Part model, mm, in its own coordinate system. A direction names the side the tool comes from. Round coordinates to 2 decimals unless told otherwise and drop trailing zeros. Loops run counter-clockwise (first coordinate to the right, second up) from the corner with the lowest first, then second, coordinate; pieces in that order, holes last.
(1) Mould opens along X. For faces 1 (the face through (92.5, -51.5, -4.8)), 2 (the face through (-96.343, -55.072, -5.916)), 3 (the face through (96.343, 55.072, -5.916)) say: +X half, -X half, draft (parallel to the pull), parting line (faces both ways), or undercut.
(2) Tool access for faces 4 (the face through (-74, -38, -11.4)), 5 (the face through (57.83, -29.62, -11.7)), 6 (the face through (96.172, -55.243, -5.916)): list every direction of +Z, -Z, +X, -X, +Y, -Y with a clear straight run to the whole face (end or side of a thin tool).
(3) Flat gauge pins, fed straight in: pin 1 (0.5 mm diameter, centred on y = -48, z = -12, fed in from -X); pin 2 (7.5 mm diameter, centred on x = -76.5, y = -40, fed in from +Z). Where does each tip first touch, or does it go through?
(4) Cut at D-D on y = 33.8. List the corners of the cut face in (x, z) (3 decimals), then the cut area to 3 significant figures.
(5) Cut at A-A on y = 9.5. List the corners of the cut face in (x, z) (3 decimals).
(6) Cut at B-B on z = -4.75. List the corners of the cut face in (x, y).
(7) Probe probe 1 along X at (y, z) = (-16.5, -5); probe 2 along Y at (x, z) = (-63.1, -11.6) (3 decimals); probe 3 along Y at (x, z) = (83, -8). List the from-to ranges inside material, lowest first.
(8) Cut at C-C on x = -33.5. List the corners of the cut face in (y, z) (3 decimals).
Autodesk Inventor part; units mm, degrees
ref_plane "YZ Plane" through (0, 0, 0) normal (1, 0, 0) x (0, 1, 0)
ref_plane "XZ Plane" through (0, 0, 0) normal (0, 1, 0) x (-1, 0, 0)
ref_plane "XY Plane" through (0, 0, 0) normal (0, 0, 1) x (1, 0, 0)
sketch "Sketch1" plane through (0, 0, 0) normal (0, 0, 1) x (1, 0, 0)
  line L0 (77.5, 43.5) -> (77.5, -43.5)
  line L1 (77.5, -43.5) -> (-77.5, -43.5)
  line L2 (-77.5, -43.5) -> (-77.5, 43.5)
  line L3 (-77.5, 43.5) -> (77.5, 43.5)
  line L4 (85.48, 55.38) -> (-85.48, 55.38)
  arc A0 (-85.48, 55.38) -> (-96.48, 44.38) centre (-85.48, 44.38) ccw
  line L5 (-96.48, 44.38) -> (-96.48, -44.38)
  arc A1 (-96.48, -44.38) -> (-85.48, -55.38) centre (-85.48, -44.38) ccw
  line L6 (-85.48, -55.38) -> (85.48, -55.38)
  arc A2 (85.48, -55.38) -> (96.48, -44.38) centre (85.48, -44.38) ccw
  line L7 (96.48, -44.38) -> (96.48, 44.38)
  arc A3 (96.48, 44.38) -> (85.48, 55.38) centre (85.48, 44.38) ccw
  line L8 (-88.48, 58.38) -> (88.48, 58.38)
  line L9 (99.48, 47.38) -> (99.48, -47.38)
  line L10 (88.48, -58.38) -> (-88.48, -58.38)
  line L11 (-99.48, -47.38) -> (-99.48, 47.38)
  arc A4 (-88.48, 58.38) -> (-99.48, 47.38) centre (-88.48, 47.38) ccw
  arc A5 (99.48, 47.38) -> (88.48, 58.38) centre (88.48, 47.38) ccw
  arc A6 (88.48, -58.38) -> (99.48, -47.38) centre (88.48, -47.38) ccw
  arc A7 (-99.48, -47.38) -> (-88.48, -58.38) centre (-88.48, -47.38) ccw
  point P0 (0, 0)
  dimension "d0" = 3
  dimension "d1" = 3
  dimension "d2" = 3
  dimension "d3" = 3
  dimension "d4" = 11
  dimension "d5" = 11
extrude "Extrusion1" add sketch "Sketch1" against normal blind 12 contours L0 L1 L2 L3 | A3 L7 A2 L6 A1 L5 A0 L4 | L8 A5 L9 A6 L10 A7 L11 A4
sketch "Sketch2" plane through (0, 0, 0) normal (0, 0, 1) x (1, 0, 0)
  line L0 (-88.48, 58.38) -> (88.48, 58.38)
  arc A0 (-88.48, 58.38) -> (-99.48, 47.38) centre (-88.48, 47.38) ccw
  line L1 (-99.48, -47.38) -> (-99.48, 47.38)
  arc A1 (-99.48, -47.38) -> (-88.48, -58.38) centre (-88.48, -47.38) ccw
  line L2 (88.48, -58.38) -> (-88.48, -58.38)
  arc A2 (88.48, -58.38) -> (99.48, -47.38) centre (88.48, -47.38) ccw
  line L3 (99.48, 47.38) -> (99.48, -47.38)
  arc A3 (99.48, 47.38) -> (88.48, 58.38) centre (88.48, 47.38) ccw
  line L4 (77.5, 43.5) -> (77.5, -43.5)
  line L5 (77.5, -43.5) -> (-77.5, -43.5)
  line L6 (-77.5, -43.5) -> (-77.5, 43.5)
  line L7 (-77.5, 43.5) -> (77.5, 43.5)
  line L8 (85.48, 55.38) -> (-85.48, 55.38)
  arc A4 (-85.48, 55.38) -> (-96.48, 44.38) centre (-85.48, 44.38) ccw
  line L9 (-96.48, 44.38) -> (-96.48, -44.38)
  arc A5 (-96.48, -44.38) -> (-85.48, -55.38) centre (-85.48, -44.38) ccw
  line L10 (-85.48, -55.38) -> (85.48, -55.38)
  arc A6 (85.48, -55.38) -> (96.48, -44.38) centre (85.48, -44.38) ccw
  line L11 (96.48, -44.38) -> (96.48, 44.38)
  arc A7 (96.48, 44.38) -> (85.48, 55.38) centre (85.48, 44.38) ccw
  arc A8 (-85.48, 56.38) -> (-97.48, 44.38) centre (-85.48, 44.38) ccw
  line L12 (-85.48, 56.38) -> (85.48, 56.38)
  arc A9 (97.48, 44.38) -> (85.48, 56.38) centre (85.48, 44.38) ccw
  line L13 (97.48, 44.38) -> (97.48, -44.38)
  arc A10 (85.48, -56.38) -> (97.48, -44.38) centre (85.48, -44.38) ccw
  line L14 (85.48, -56.38) -> (-85.48, -56.38)
  arc A11 (-97.48, -44.38) -> (-85.48, -56.38) centre (-85.48, -44.38) ccw
  line L15 (-97.48, -44.38) -> (-97.48, 44.38)
  point P0 (0, 0)
  dimension "d8" = 1
extrude "Extrusion2" cut sketch "Sketch2" against normal blind 1.5 contours L4 L5 L6 L7 | A7 L11 A6 L10 A5 L9 A4 L8 | L12 A9 L13 A10 L14 A11 L15 A8
sketch "Sketch3" plane through (0, 0, -1.5) normal (0, 0, 1) x (1, 0, 0)
  arc A0 (-85.48, 56.38) -> (-97.48, 44.38) centre (-85.48, 44.38) ccw
  line L0 (-97.48, -44.38) -> (-97.48, 44.38)
  arc A1 (-97.48, -44.38) -> (-85.48, -56.38) centre (-85.48, -44.38) ccw
  line L1 (85.48, -56.38) -> (-85.48, -56.38)
  arc A2 (85.48, -56.38) -> (97.48, -44.38) centre (85.48, -44.38) ccw
  line L2 (97.48, 44.38) -> (97.48, -44.38)
  arc A3 (97.48, 44.38) -> (85.48, 56.38) centre (85.48, 44.38) ccw
  line L3 (-85.48, 56.38) -> (85.48, 56.38)
  arc A4 (-85.48, 54.38) -> (-95.48, 44.38) centre (-85.48, 44.38) ccw
  line L4 (-85.48, 54.38) -> (85.48, 54.38)
  arc A5 (95.48, 44.38) -> (85.48, 54.38) centre (85.48, 44.38) ccw
  line L5 (95.48, 44.38) -> (95.48, -44.38)
  arc A6 (85.48, -54.38) -> (95.48, -44.38) centre (85.48, -44.38) ccw
  line L6 (85.48, -54.38) -> (-85.48, -54.38)
  arc A7 (-95.48, -44.38) -> (-85.48, -54.38) centre (-85.48, -44.38) ccw
  line L7 (-95.48, -44.38) -> (-95.48, 44.38)
  point P0 (0, 0)
  dimension "d11" = 2
extrude "Extrusion3" cut sketch "Sketch3" against normal blind 9.9 contours L4 A5 L5 A6 L6 A7 L7 A4
fillet "Fillet1" radius 3.175 8 edges at (92.5511, 51.4511, -11.4) (95.48, 0, -11.4) (92.5511, -51.4511, -11.4) (0, -54.38, -11.4) (-92.5511, -51.4511, -11.4) (-95.48, 0, -11.4) (-92.5511, 51.4511, -11.4) (0, 54.38, -11.4)
sketch "Sketch5" plane through (0, 0, -12) normal (0, 0, -1) x (-1, 0, 0)
  arc A0 (-85.48, 51.205) -> (-92.305, 44.38) centre (-85.48, 44.38) ccw
  line L0 (85.48, 51.205) -> (-85.48, 51.205)
  arc A1 (92.305, 44.38) -> (85.48, 51.205) centre (85.48, 44.38) ccw
  line L1 (92.305, -44.38) -> (92.305, 44.38)
  arc A2 (85.48, -51.205) -> (92.305, -44.38) centre (85.48, -44.38) ccw
  line L2 (-85.48, -51.205) -> (85.48, -51.205)
  arc A3 (-92.305, -44.38) -> (-85.48, -51.205) centre (-85.48, -44.38) ccw
  line L3 (-92.305, 44.38) -> (-92.305, -44.38)
  circle A4 centre (-63.1, 33.8) radius 1.5
  circle A5 centre (-63.1, -31.85) radius 1.5
  circle A6 centre (63.1, -31.85) radius 1.5
  circle A7 centre (63.1, 33.8) radius 1.5
  circle A8 centre (-63.1, 33.8) radius 1.905
  circle A9 centre (63.1, 33.8) radius 1.905
  circle A10 centre (63.1, -31.85) radius 1.905
  circle A11 centre (-63.1, -31.85) radius 1.905
  line L4 (-54.205, 51.205) -> (-54.205, 38.505)
  line L5 (-66.905, 25.805) -> (-92.305, 25.805)
  arc A12 (-66.905, 25.805) -> (-54.205, 38.505) centre (-66.905, 38.505) ccw
  line L6 (0, 51.205) -> (0, -51.205)
  line L7 (-92.305, 0) -> (92.305, 0)
  line L8 (54.205, 51.205) -> (54.205, 38.505)
  line L9 (66.905, 25.805) -> (92.305, 25.805)
  arc A13 (54.205, 38.505) -> (66.905, 25.805) centre (66.905, 38.505) ccw
  line L10 (-54.205, -51.205) -> (-54.205, -38.505)
  line L11 (-66.905, -25.805) -> (-92.305, -25.805)
  arc A14 (-54.205, -38.505) -> (-66.905, -25.805) centre (-66.905, -38.505) ccw
  line L12 (54.205, -51.205) -> (54.205, -38.505)
  arc A15 (66.905, -25.805) -> (54.205, -38.505) centre (66.905, -38.505) ccw
  line L13 (66.905, -25.805) -> (92.305, -25.805)
  line L14 (-54.205, 51.205) -> (54.205, 51.205)
  line L15 (92.305, 25.805) -> (92.305, -25.805)
  line L16 (54.205, -51.205) -> (-54.205, -51.205)
  line L17 (-92.305, -25.805) -> (-92.305, 25.805)
  point P0 (0, 0)
  dimension "d38" = 3.81
  dimension "d39" = 3.81
  dimension "d40" = 3.81
  dimension "d41" = 3.81
  dimension "d51" = 12.7
  dimension "d52" = 25.4
  dimension "d53" = 38.1
extrude "Extrusion4" cut sketch "Sketch5" against normal through all contours L0 L6 L7 L3 L5 A12 L4 | L0 L8 A13 L9 L1 L7 L6 | L7 L6 L2 L10 A14 L11 L3 | L7 L1 L13 A15 L12 L2 L6 | A4 | A5 | A6 | A7 | A8 | A9 | A10 | A11
equation "\"d1\" = d0"
equation "\"d2\" = d0"
equation "\"d3\" = d0"
equation "\"d4\" = d5"
equation "\"d39\" = d38"
equation "\"d40\" = d38"
equation "\"d41\" = d38"
properties part number "Hub Enclosure Front"
Final values:
1. face 1: undercut
1. face 2: -X half
1. face 3: +X half
2. face 4: +Z
2. face 5: +Z, -Z
2. face 6: +Z, -Z, +X, -Y
3. pin 1: stops at x = -99.47
3. pin 2: stops at z = -11.4
4. outline: (-99.48, -12) - (-65.005, -12) - (-65.005, -11.4) - (-92.305, -11.4) arc R3.175 cw to (-95.48, -8.225) - (-95.48, -1.5) - (-97.48, -1.5) - (-97.48, 0) - (-99.48, 0) - close; (-61.195, -12) - (-55.109, -12) - (-55.109, -11.4) - (-61.195, -11.4) - close; (55.109, -12) - (61.195, -12) - (61.195, -11.4) - (55.109, -11.4) - close; (65.005, -12) - (99.48, -12) - (99.48, 0) - (97.48, 0) - (97.48, -1.5) - (95.48, -1.5) - (95.48, -8.225) arc R3.175 cw to (92.305, -11.4) - (65.005, -11.4) - close
4. area: 138 mm2
5. outline: (-99.48, -12) - (-92.305, -12) - (-92.305, -11.4) arc R3.175 cw to (-95.48, -8.225) - (-95.48, -1.5) - (-97.48, -1.5) - (-97.48, 0) - (-99.48, 0) - close; (92.305, -12) - (99.48, -12) - (99.48, 0) - (97.48, 0) - (97.48, -1.5) - (95.48, -1.5) - (95.48, -8.225) arc R3.175 cw to (92.305, -11.4) - close
6. outline: (-99.48, -47.38) arc R11 ccw to (-88.48, -58.38) - (88.48, -58.38) arc R11 ccw to (99.48, -47.38) - (99.48, 47.38) arc R11 ccw to (88.48, 58.38) - (-88.48, 58.38) arc R11 ccw to (-99.48, 47.38) - close; hole (-95.48, -44.38) arc R10 ccw to (-85.48, -54.38) - (85.48, -54.38) arc R10 ccw to (95.48, -44.38) - (95.48, 44.38) arc R10 ccw to (85.48, 54.38) - (-85.48, 54.38) arc R10 ccw to (-95.48, 44.38) - close
7. probe 1: x = -99.48 to -95.48, 95.48 to 99.48
7. probe 2: y = -58.38 to -33.755, -29.945 to -26.388, 26.388 to 31.895, 35.705 to 58.38
7. probe 3: y = -58.38 to -54.38, 54.38 to 58.38
8. outline: (-58.38, -12) - (-51.205, -12) - (-51.205, -11.4) arc R3.175 cw to (-54.38, -8.225) - (-54.38, -1.5) - (-56.38, -1.5) - (-56.38, 0) - (-58.38, 0) - close; (51.205, -12) - (58.38, -12) - (58.38, 0) - (56.38, 0) - (56.38, -1.5) - (54.38, -1.5) - (54.38, -8.225) arc R3.175 cw to (51.205, -11.4) - close
